The model under review builds one solid part; all positions refer to its coordinate system, in mm. A direction names the side the tool comes from. Give positions to 0.01 mm unless a question says otherwise; leave off trailing zeros. Loops run counter-clockwise (first coordinate to the right, second up) from the corner with the lowest first, then second, coordinate; pieces in that order, holes last. Notation, with made-up numbers: M 32.25,38 L 58.25,38 A31 cw 58.25,73 Z; hole C 39.5,16.5 d3. An arc over 180 degrees is marked long. Return JSON: item names as keys, results as strings.
Autodesk Inventor part; units mm, degrees
ref_plane "YZ Plane" through (0, 0, 0) normal (1, 0, 0) x (0, 1, 0)
ref_plane "XZ Plane" through (0, 0, 0) normal (0, 1, 0) x (-1, 0, 0)
ref_plane "XY Plane" through (0, 0, 0) normal (0, 0, 1) x (1, 0, 0)
sketch "Sketch1" plane through (0, 0, 0) normal (0, 0, 1) x (1, 0, 0)
  line L0 (0, 0) -> (76.2, 0)
  line L1 (76.2, 0) -> (76.2, 25.4)
  line L2 (76.2, 25.4) -> (25.4, 25.4)
  line L3 (0, 25.4) -> (0, 0)
  line L4 (0, 0) -> (25.4, 0)
  line L5 (25.4, 25.4) -> (25.4, 76.2)
  line L6 (25.4, 76.2) -> (0, 76.2)
  line L7 (0, 76.2) -> (0, 0)
  line L8 (12.7, 76.2) -> (12.7, 63.5) construction
  line L9 (12.7, 63.5) -> (12.7, 38.1) construction
  line L10 (12.7, 38.1) -> (12.7, 12.7) construction
  line L11 (12.7, 12.7) -> (38.1, 12.7) construction
  line L12 (38.1, 12.7) -> (63.5, 12.7) construction
  circle A0 centre (12.7, 63.5) radius 2.5797
  circle A1 centre (12.7, 38.1) radius 2.5797
  circle A2 centre (12.7, 12.7) radius 2.5797
  circle A3 centre (38.1, 12.7) radius 2.5797
  circle A4 centre (63.5, 12.7) radius 2.5797
  dimension "d0" = 76.2
  dimension "d1" = 25.4
  dimension "d2" = 25.4
  dimension "d3" = 76.2
  dimension "d4" = 12.7
  dimension "d5" = 25.4
  dimension "d6" = 25.4
  dimension "d7" = 25.4
  dimension "d8" = 25.4
  dimension "d9" = 5.1594
extrude "Extrusion1" add sketch "Sketch1" along normal blind 3.175
sketch "Sketch2" plane through (0, 0, 3.175) normal (0, 0, 1) x (1, 0, 0)
  circle A0 centre (12.7, 63.5) radius 2.5797 construction
  line L0 (12.7, 63.5) -> (12.7, 88.9) construction
  line L1 (12.7, 88.9) -> (12.7, 114.3) construction
  circle A1 centre (63.5, 12.7) radius 2.5797 construction
  line L2 (63.5, 12.7) -> (88.9, 12.7) construction
  line L3 (88.9, 12.7) -> (114.3, 12.7) construction
  circle A2 centre (88.9, 12.7) radius 2.5797
  circle A3 centre (114.3, 12.7) radius 2.5797
  circle A4 centre (12.7, 88.9) radius 2.5797
  circle A5 centre (12.7, 114.3) radius 2.5797
  line L4 (0, 76.2) -> (0, 0)
  line L5 (0, 76.2) -> (0, 127)
  line L6 (0, 127) -> (25.4, 127)
  line L7 (25.4, 25.4) -> (25.4, 76.2)
  line L8 (25.4, 127) -> (25.4, 76.2)
  line L9 (25.4, 76.2) -> (0, 76.2)
  line L10 (76.2, 0) -> (76.2, 25.4)
  line L11 (76.2, 25.4) -> (76.2, 0)
  line L12 (76.2, 0) -> (127, 0)
  line L13 (127, 0) -> (127, 25.4)
  line L14 (127, 25.4) -> (76.2, 25.4)
  dimension "d12" = 25.4
  dimension "d13" = 25.4
  dimension "d14" = 25.4
  dimension "d15" = 25.4
  dimension "d16" = 50.8
  dimension "d17" = 25.4
  dimension "d18" = 50.8
extrude "Extrusion2" add sketch "Sketch2" against normal blind 3.175
properties part number "L gusset"
1) Consider section A-A on y = 114.3. Write out the cut boundary in (x, z) (3 decimals).
From the geometry:
{"outline": "M 0,0 L 10.12,0 L 10.12,3.175 L 0,3.175 Z; M 15.28,0 L 25.4,0 L 25.4,3.175 L 15.28,3.175 Z"}
2) The part is to be moulded in two halves that separate along Y. For faces 1 (the face through (25.4, 75, 2)), 2 (the face through (13, 127, 2)), 3 (the face through (63, 0, 2)), 4 (the face through (12.364, 91.458, 1.61)), say which applies: released by +Y, released by -Y, zero draft, split by the parting line, or undercut.
From the geometry:
{"face 1": "zero draft", "face 2": "released by +Y", "face 3": "released by -Y", "face 4": "undercut"}
3) Insertion check: pin 1 (1 mm diameter, centred on y = 48, z = 2.5, fed in from +X); pin 2 (1 mm diameter, centred on x = 75, z = 2, fed in from +Y). Each pin has a flat end and moves straight along its axis. Give the tip position at first contact, or say it passes through.
From the geometry:
{"pin 1": "x = 25.4", "pin 2": "y = 25.4"}
4) Consider section C-C on z = 1. Count the separate pieces of the cut face and the enclosed holes in it, then the cut area to 3 significant figures.
From the geometry:
{"separate pieces": "1", "enclosed holes": "9", "area": "5,620 mm²"}
5) Tool access review of faces 5 (the face through (77, 25.4, 2)), 6 (the face through (34, 22, 3.175)): name each direction out of +Z, -Z, +X, -X, +Y, -Y from which nothing blocks a thin tool from reaching the whole face with its end or side.
From the geometry:
{"face 5": "+Z, -Z, +X, +Y", "face 6": "+Z, +X, -X, +Y, -Y"}
6) Consider section D-D on y = 12.7. Write out the cut boundary in (x, z) (3 decimals), then the cut area to 3 significant figures.
From the geometry:
{"outline": "M 0,0 L 10.12,0 L 10.12,3.175 L 0,3.175 Z; M 15.28,0 L 35.52,0 L 35.52,3.175 L 15.28,3.175 Z; M 40.68,0 L 60.92,0 L 60.92,3.175 L 40.68,3.175 Z; M 66.08,0 L 86.32,0 L 86.32,3.175 L 66.08,3.175 Z; M 91.48,0 L 111.72,0 L 111.72,3.175 L 91.48,3.175 Z; M 116.88,0 L 127,0 L 127,3.175 L 116.88,3.175 Z", "area": "321 mm²"}
7) Wall thickness on L1, parallel to Y at x = 12.7, z = 1.35; L2, parallel to Y at x = 114.3, z = 0.8; L3, parallel to Y at x = 96, z = 1.45: over which ranges is each line inside the solid? List them lowest first. Write a range as from..to.
From the geometry:
{"L1": "0..10.12, 15.28..35.52, 40.68..60.92, 66.08..86.32, 91.48..111.72, 116.88..127", "L2": "0..10.12, 15.28..25.4", "L3": "0..25.4"}
